Autodesk Inventor part; units mm, degrees
ref_plane "Piano di lavoro1" through (0, 13.85, 0) normal (0, 1, 0) x (1, 0, 0)
ref_plane "Piano di lavoro2" through (0, -10.75, 0) normal (0, -1, 0) x (1, 0, 0)
ref_plane "YZ Plane" through (0, 0, 0) normal (1, 0, 0) x (0, 1, 0)
sketch "Schizzo1" plane through (0, 0, 0) normal (0, 1, 0) x (-1, 0, 0)
  line L0 (-8.85, -17.84) -> (8.95, -17.84)
  line L1 (8.95, -17.84) -> (8.95, 17.78)
  line L2 (8.95, 17.78) -> (-8.85, 17.78)
  line L3 (-8.85, 17.78) -> (-8.85, -17.84)
  line L4 (-8.85, 17.78) -> (8.95, -17.84) construction
  line L5 (8.95, 17.78) -> (-8.85, -17.84) construction
  line L6 (8.95, 16.48) -> (-8.95, 16.48) construction
  line L7 (-7.6, 17.78) -> (-7.6, -17.84) construction
  circle A0 centre (-7.6, 16.48) radius 0.425
  circle A1 centre (-7.6, 13.94) radius 0.425
  circle A2 centre (-7.6, 11.4) radius 0.425
  circle A3 centre (-7.6, 8.86) radius 0.425
  circle A4 centre (-7.6, 6.32) radius 0.425
  circle A5 centre (-7.6, 3.78) radius 0.425
  circle A6 centre (-7.6, 1.24) radius 0.425
  circle A7 centre (-7.6, -1.3) radius 0.425
  circle A8 centre (-7.6, -3.84) radius 0.425
  circle A9 centre (-7.6, -6.38) radius 0.425
  circle A10 centre (-7.6, -8.92) radius 0.425
  circle A11 centre (-7.6, -11.46) radius 0.425
  circle A12 centre (-7.6, -14) radius 0.425
  circle A13 centre (-7.6, -16.54) radius 0.425
  circle A14 centre (-5.06, 16.48) radius 0.425
  circle A15 centre (-2.52, 16.48) radius 0.425
  circle A16 centre (0.02, 16.48) radius 0.425
  circle A17 centre (2.56, 16.48) radius 0.425
  circle A18 centre (5.1, 16.48) radius 0.425
  circle A19 centre (7.64, 16.48) radius 0.425
  circle A20 centre (7.64, 13.94) radius 0.425
  circle A21 centre (7.64, 11.4) radius 0.425
  circle A22 centre (7.64, 8.86) radius 0.425
  circle A23 centre (7.64, 6.32) radius 0.425
  circle A24 centre (7.64, 3.78) radius 0.425
  circle A25 centre (7.64, 1.24) radius 0.425
  circle A26 centre (7.64, -1.3) radius 0.425
  circle A27 centre (7.64, -3.84) radius 0.425
  circle A28 centre (7.64, -6.38) radius 0.425
  circle A29 centre (7.64, -8.92) radius 0.425
  circle A30 centre (7.64, -11.46) radius 0.425
  circle A31 centre (7.64, -14) radius 0.425
  circle A32 centre (7.64, -16.54) radius 0.425
  circle A33 centre (-5.06, -14) radius 0.425
  circle A34 centre (-5.06, -8.92) radius 0.425
  circle A35 centre (-5.06, -6.38) radius 0.425
  circle A36 centre (-5.06, -3.84) radius 0.425
  point P0 (0, 0)
  point P1 (0.05, -0.03)
  dimension "d0" = 17.8
  dimension "d1" = 35.62
  dimension "d4" = 1.3
  dimension "d5" = 1.25
  dimension "d6" = 0.85
  dimension "d9" = 2.54
  dimension "d16" = 2.54
  dimension "d23" = 2.54
  dimension "d79" = 2.54
extrude "Estrusione2" add sketch "Schizzo1" along normal blind 1.6
fillet "Raccordo1" radius 0.2 12 edges at (-0.05, 0, 17.78) (-0.05, 1.6, 17.78) (8.85, 0.8, 17.78) (8.85, 0, -0.03) (8.85, 1.6, -0.03) (8.85, 0.8, -17.84) (-0.05, 0, -17.84) (-8.95, 0, -0.03) (-8.95, 0.8, -17.84) (-8.95, 0.8, 17.78) (-8.95, 1.6, -0.03) (-0.05, 1.6, -17.84)
ref_plane "Piano di lavoro1" through (0, 13.85, 0) normal (0, 1, 0) x (1, 0, 0)
sketch "Schizzo2" plane through (0, 13.85, 0) normal (0, 1, 0) x (1, 0, 0)
  line L0 (8.8439, 19.3342) -> (8.8439, -17.791) construction
  line L1 (8.8439, -17.791) -> (-8.9298, -17.791) construction
  line L2 (-8.9298, -17.791) -> (-8.9298, 19.3342) construction
  line L3 (-8.9298, 19.3342) -> (8.8439, 19.3342) construction
  point P0 (0, 0)
decal "Decalcomania1"
ref_plane "Piano di lavoro2" through (0, -10.75, 0) normal (0, -1, 0) x (1, 0, 0)
sketch "Schizzo3" plane through (0, -10.75, 0) normal (0, -1, 0) x (1, 0, 0)
  line L0 (9.0107, 17.7535) -> (9.0107, -19.0765) construction
  line L1 (9.0107, -19.0765) -> (-8.7138, -19.0765) construction
  line L2 (-8.7138, -19.0765) -> (-8.7138, 17.7535) construction
  line L3 (-8.7138, 17.7535) -> (9.0107, 17.7535) construction
  point P0 (0, 0)
decal "Decalcomania2"
sketch "Schizzo4" plane through (0, 1.6, 0) normal (0, 1, 0) x (1, 0, 0)
  circle A0 centre (7.6, 11.46) radius 0.425
sketch "Schizzo5" plane through (0, 1.6, 0) normal (0, 1, 0) x (1, 0, 0)
  circle A0 centre (7.6, -1.24) radius 0.425
sketch "Schizzo6" plane through (0, 1.6, 0) normal (0, 1, 0) x (1, 0, 0)
  circle A0 centre (7.6, -3.78) radius 0.425
sketch "Schizzo7" plane through (0, 1.6, 0) normal (0, 1, 0) x (1, 0, 0)
  circle A0 centre (-7.64, 16.54) radius 0.425
sketch "Schizzo8" plane through (0, 1.6, 0) normal (0, 1, 0) x (1, 0, 0)
  circle A0 centre (-7.64, 14) radius 0.425
sketch "Schizzo9" plane through (0, 1.6, 0) normal (0, 1, 0) x (1, 0, 0)
  circle A0 centre (-7.64, 11.46) radius 0.425
sketch "Sketch10" plane through (0, 0, 0) normal (0, -1, 0) x (1, 0, 0)
  circle A0 centre (7.6, -11.46) radius 0.425
sketch "Schizzo11" plane through (0, 0, 0) normal (0, -1, 0) x (1, 0, 0)
  circle A0 centre (-7.64, -16.54) radius 0.425
sketch "Schizzo12" plane through (0, 1.6, 0) normal (0, 1, 0) x (1, 0, 0)
  circle A0 centre (-7.64, -11.4) radius 0.425
sketch "Schizzo13" plane through (0, 1.6, 0) normal (0, 1, 0) x (1, 0, 0)
  circle A0 centre (-7.64, -8.86) radius 0.425
sketch "Schizzo14" plane through (0, 0, 0) normal (0, -1, 0) x (1, 0, 0)
  circle A0 centre (7.6, 1.24) radius 0.425
sketch "Schizzo15" plane through (0, 0, 0) normal (0, -1, 0) x (1, 0, 0)
  circle A0 centre (7.6, 3.78) radius 0.425
properties part number "101" material "Plastica ABS"
Check sheet for the modelled part. Datum: model origin and axes. Units: mm. Coordinates: 2 decimals unless noted, no trailing zeros. Loops run counter-clockwise (first coordinate to the right, second up) from the corner with the lowest first, then second, coordinate; pieces in that order, holes last. Notation, with made-up numbers: (1, -37) -> (55, -37) arc R20 cw to (55, -27) -> close; hole circle Ø5 at (-38, -31). An arc over 180 degrees is marked (long way). Answer in a Markdown table with one row per item.
1. Sectioned sample at C-C, the plane z = 6.32. Record the boundary of the cut face in (x, y) (3 decimals), then the cut area to 3 significant figures.
Check values:
| item | result |
|---|---|
| outline | (-8.95, 0.2) arc R0.2 ccw to (-8.75, 0) -> (-8.065, 0) -> (-8.065, 1.6) -> (-8.75, 1.6) arc R0.2 ccw to (-8.95, 1.4) -> close; (-7.215, 0) -> (7.175, 0) -> (7.175, 1.6) -> (-7.215, 1.6) -> close; (8.025, 0) -> (8.65, 0) arc R0.2 ccw to (8.85, 0.2) -> (8.85, 1.4) arc R0.2 ccw to (8.65, 1.6) -> (8.025, 1.6) -> close |
| area | 25.7 mm2 |
2. Sectioned sample at A-A, the plane z = -14. Record the boundary of the cut face in (x, y) (3 decimals).
Check values:
| item | result |
|---|---|
| outline | (-8.95, 0.2) arc R0.2 ccw to (-8.75, 0) -> (-8.065, 0) -> (-8.065, 1.6) -> (-8.75, 1.6) arc R0.2 ccw to (-8.95, 1.4) -> close; (-7.215, 0) -> (4.635, 0) -> (4.635, 1.6) -> (-7.215, 1.6) -> close; (5.485, 0) -> (7.175, 0) -> (7.175, 1.6) -> (5.485, 1.6) -> close; (8.025, 0) -> (8.65, 0) arc R0.2 ccw to (8.85, 0.2) -> (8.85, 1.4) arc R0.2 ccw to (8.65, 1.6) -> (8.025, 1.6) -> close |
3. Release check for a two-part mould opening along X. For faces 1 (the face through (0, 1, -17.84)), 2 (the face through (5.485, 0.789, -6.399)), 3 (the face through (8.85, 1, 0)) record: released by +X, released by -X, zero draft, split by the parting line, or undercut.
Check values:
| item | result |
|---|---|
| face 1 | zero draft |
| face 2 | undercut |
| face 3 | released by +X |
4. Material ranges on line 1 along X through (y, z) = (0.7, -9); line 2 along X through (y, z) = (0.4, -16.54) (3 decimals); line 3 along Z through (x, y) = (2.5, 0.95), recorded low to high. Write a range as [from, to].
Check values:
| item | result |
|---|---|
| line 1 | x = [-8.95, -8.06], [-7.22, 4.64], [5.48, 7.18], [8.02, 8.85] |
| line 2 | x = [-8.95, -8.065], [-7.215, 7.175], [8.025, 8.85] |
| line 3 | z = [-17.84, 16.06], [16.9, 17.78] |
5. Sectioned sample at B-B, the plane x = 2.52. Record the boundary of the cut face in (y, z) (3 decimals).
Check values:
| item | result |
|---|---|
| outline | (0, -17.64) arc R0.2 ccw to (0.2, -17.84) -> (1.4, -17.84) arc R0.2 ccw to (1.6, -17.64) -> (1.6, 16.055) -> (0, 16.055) -> close; (0, 16.905) -> (1.6, 16.905) -> (1.6, 17.58) arc R0.2 ccw to (1.4, 17.78) -> (0.2, 17.78) arc R0.2 ccw to (0, 17.58) -> close |
6. Sectioned sample at D-D, the plane y = 1.1. Give the number of separate pieces and of enclosed holes in the cut face, then the cut area to 3 significant figures.
Check values:
| item | result |
|---|---|
| separate pieces | 1 |
| enclosed holes | 37 |
| area | 613 mm2 |
